Drawing for the job (mm, zero at the part's lowest x, y, z). Round coordinates to 2 decimals unless told otherwise and drop trailing zeros. Loops run counter-clockwise (first coordinate to the right, second up) from the corner with the lowest first, then second, coordinate; pieces in that order, holes last. Notation, with made-up numbers: M 45,24.5 L 72,24.5 A17 cw 72,35.5 Z; hole C 62.25,-31.5 d6. An arc over 180 degrees is marked long. Use a Markdown table: item, result. Add a question column.
Q1. Pin check, flat tips, straight feed: pin 1 (2 mm diameter, centred on x = 58.5, y = 29, fed in from +Z); pin 2 (2.5 mm diameter, centred on y = 36, z = 2.5, fed in from +X). Stop position of each tip, or through.
Q2. Probe line 1 (X direction, y = 6.5, z = 3) (1 decimal); line 2 (X direction, y = 44, z = 4.3); line 3 (Y direction, x = 78, z = 2.85). List the from-to ranges inside material, lowest first. Write a range as from..to.
Q3. Cut at B-B (z = 0.85). State how many separate pieces and enclosed holes the cut face has, plus the area to 3 significant figures.
Q4. Cut at C-C (x = 76). Give the cut face in (y, z).
Q5. Cut at A-A (y = 6.35). Give the cut face in (x, z) (1 decimal), plus the area to 3 significant figures.
Q6. Mould opens along X. For the marked faces 1 and 2 say: +X half, -X half, draft (parallel to the pull), parting line (faces both ways), or undercut.
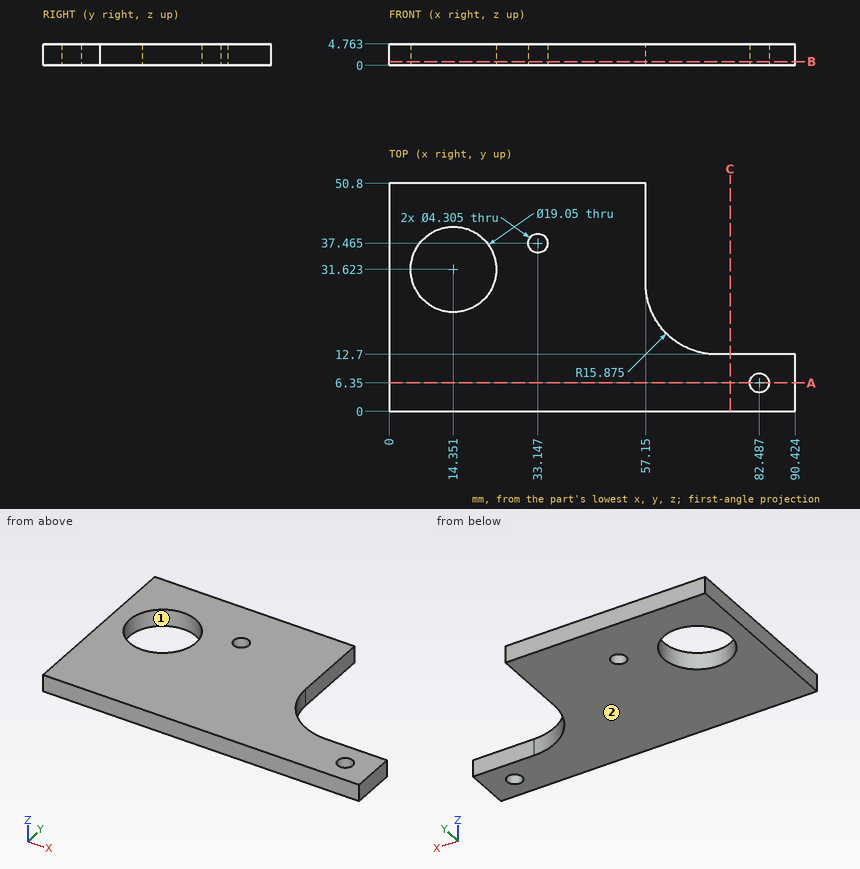
Checked values:
| question | item | result |
|---|---|---|
| 1 | pin 1 | passes through |
| 1 | pin 2 | stops at x = 57.15 |
| 2 | line 1 | x = 0..80.3, 84.6..90.4 |
| 2 | line 2 | x = 0..57.15 |
| 2 | line 3 | y = 0..12.7 |
| 3 | separate pieces | 1 |
| 3 | enclosed holes | 3 |
| 3 | area | 3,070 mm^2 |
| 4 | outline | M 0,0 L 12.7,0 L 12.7,4.76 L 0,4.76 Z |
| 5 | outline | M 0,0 L 80.3,0 L 80.3,4.8 L 0,4.8 Z; M 84.6,0 L 90.4,0 L 90.4,4.8 L 84.6,4.8 Z |
| 5 | area | 410 mm^2 |
| 6 | face 1 | undercut |
| 6 | face 2 | draft |
